Read the model definition and answer for the solid it produces. Units are mm, in the model's axes. Give positions to 0.01 mm unless a question says otherwise; leave off trailing zeros. Order: outer loops, then holes, each group sorted by start corner. A loop starts at its lowest first (then second) coordinate and runs counter-clockwise, first axis right, second up. Notation, with made-up numbers: (68.5, 26) - (79.5, 26) arc R20 cw to (79.5, 55) - close; hole circle Ø11 at (36, 15.25). An arc over 180 degrees is marked (long way). Answer as CSV lines item,"result". Start each with the question number.
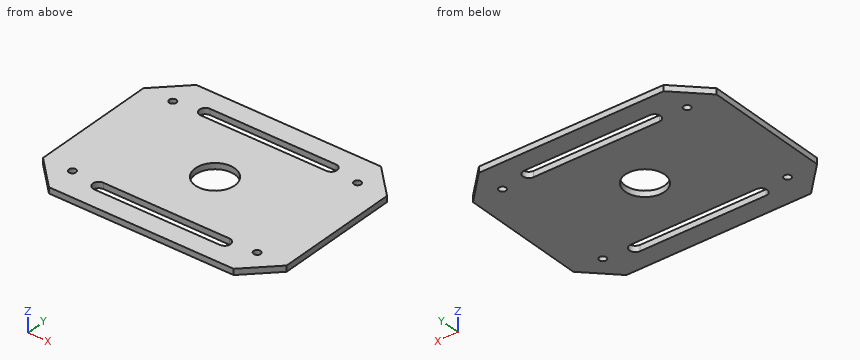
from build123d import *

# Parameters (mm, degrees)
SKETCH1_R           = 1.8
SKETCH1_R_2         = 10
BOSS_EXTRUDE1_DEPTH = 3


with BuildPart() as part:
    # Sketch1 → Boss-Extrude1 (new body)
    with BuildSketch(Plane.XY):
        Polygon((-39.957408855, -43.544565591), (-24.957408855, -28.544565591), (69.042591145, -28.544565591), (84.042591145, -43.544565591), (84.042591145, -107.544565591), (69.042591145, -122.544565591), (-24.957408855, -122.544565591), (-39.957408855, -107.544565591), align=None)
        with Locations((-24.957408855, -43.544565591)):
            Circle(SKETCH1_R, mode=Mode.SUBTRACT)
        with Locations((69.042591145, -43.544565591)):
            Circle(SKETCH1_R, mode=Mode.SUBTRACT)
        with Locations((69.042591145, -107.544565591)):
            Circle(SKETCH1_R, mode=Mode.SUBTRACT)
        with Locations((-24.957408855, -107.544565591)):
            Circle(SKETCH1_R, mode=Mode.SUBTRACT)
        with Locations((22.042591145, -75.544565591)):
            Circle(SKETCH1_R_2, mode=Mode.SUBTRACT)
        with BuildLine():
            Line((-9.957408855, -38.544565591), (54.042591145, -38.544565591))
            ThreePointArc((54.042591145, -38.544565591), (57.042591145, -41.544565591), (54.042591145, -44.544565591))
            Line((54.042591145, -44.544565591), (-9.957408855, -44.544565591))
            ThreePointArc((-9.957408855, -44.544565591), (-12.957408855, -41.544565591), (-9.957408855, -38.544565591))
        make_face(mode=Mode.SUBTRACT)
        with BuildLine():
            Line((-9.965744505, -106.544565591), (54.050926794, -106.544565591))
            ThreePointArc((54.050926794, -106.544565591), (57.050926794, -109.544565591), (54.050926794, -112.544565591))
            Line((54.050926794, -112.544565591), (-9.965744505, -112.544565591))
            ThreePointArc((-9.965744505, -112.544565591), (-12.965744505, -109.544565591), (-9.965744505, -106.544565591))
        make_face(mode=Mode.SUBTRACT)
    extrude(amount=BOSS_EXTRUDE1_DEPTH)


solid = part.part
(1) Straight lines are drawn through the part: line 1 (Y direction, x = 0.5, z = 1.7); line 2 (Y direction, x = 22.5, z = 1.1); line 3 (Y direction, x = 18.5, z = 1.85). For each, find the intervals that lie inside material, in ascending order. Write a range as [from, to].
(2) Section A-A, the plane x = -1 is taken. Write down the section's boundary in (y, z), and give its area (3 significant figures).
(3) Section C-C, the plane y = -81 is taken. Write down the section's boundary in (x, z).
(4) Section B-B, the plane x = 16 is taken. Write down the section's boundary in (y, z).
(5) A flat-ended cylindrical pin translates along its axis: pin 1 Ø3 at (x, y) = (-24.96, -43.54) entering from +Z. Find the tip coordinate at first contact, or state that the pin passes through.
(6) Section D-D, the plane z = 0.45 is taken. Write down the section's boundary in (x, y).
Checks:
1,line 1,"y = [-122.54, -112.54], [-106.54, -44.54], [-38.54, -28.54]"
1,line 2,"y = [-122.54, -112.54], [-106.54, -85.53], [-65.56, -44.54], [-38.54, -28.54]"
1,line 3,"y = [-122.54, -112.54], [-106.54, -84.9], [-66.19, -44.54], [-38.54, -28.54]"
2,outline,"(-122.54, 0) - (-112.54, 0) - (-112.54, 3) - (-122.54, 3) - close; (-106.54, 0) - (-44.54, 0) - (-44.54, 3) - (-106.54, 3) - close; (-38.54, 0) - (-28.54, 0) - (-28.54, 3) - (-38.54, 3) - close"
2,area,"246 mm²"
3,outline,"(-39.96, 0) - (13.66, 0) - (13.66, 3) - (-39.96, 3) - close; (30.42, 0) - (84.04, 0) - (84.04, 3) - (30.42, 3) - close"
4,outline,"(-122.54, 0) - (-112.54, 0) - (-112.54, 3) - (-122.54, 3) - close; (-106.54, 0) - (-83.51, 0) - (-83.51, 3) - (-106.54, 3) - close; (-67.58, 0) - (-44.54, 0) - (-44.54, 3) - (-67.58, 3) - close; (-38.54, 0) - (-28.54, 0) - (-28.54, 3) - (-38.54, 3) - close"
5,pin 1,"passes through"
6,outline,"(-39.96, -107.54) - (-24.96, -122.54) - (69.04, -122.54) - (84.04, -107.54) - (84.04, -43.54) - (69.04, -28.54) - (-24.96, -28.54) - (-39.96, -43.54) - close; hole circle Ø3.6 at (-24.96, -107.54); hole circle Ø3.6 at (-24.96, -43.54); hole (-9.97, -112.54) - (54.05, -112.54) arc R3 ccw to (54.05, -106.54) - (-9.97, -106.54) arc R3 ccw to start; hole (-9.96, -44.54) - (54.04, -44.54) arc R3 ccw to (54.04, -38.54) - (-9.96, -38.54) arc R3 ccw to start; hole circle Ø20 at (22.04, -75.54); hole circle Ø3.6 at (69.04, -107.54); hole circle Ø3.6 at (69.04, -43.54)"
